```python
from build123d import *

# Parameters (mm, degrees)
F1_DEPTH = 1
F2_DEPTH = 13


with BuildPart() as f1:
    # F0 (on Top) → F1 (new body)
    with BuildSketch(Plane.XY):
        Polygon((2.864766, 10.75), (-2.864766, 10.75), (-5.25, 8.360261), (-5.25, -10.75), (5.25, -10.75), (5.25, 8.360261), align=None)
        Polygon((-4.25, 7.9466), (-2.45, 9.75), (2.45, 9.75), (4.25, 7.9466), (4.25, -9.75), (-4.25, -9.75), align=None, mode=Mode.SUBTRACT)
        Polygon((2.45, 9.75), (-2.45, 9.75), (-4.25, 7.9466), (-4.25, -9.75), (4.25, -9.75), (4.25, 7.9466), align=None)
    extrude(amount=F1_DEPTH)

    # F0 (on Top) → F2 (join)
    with BuildSketch(Plane.XY):
        Polygon((2.864766, 10.75), (-2.864766, 10.75), (-5.25, 8.360261), (-5.25, -10.75), (5.25, -10.75), (5.25, 8.360261), align=None)
        Polygon((-4.25, 7.9466), (-2.45, 9.75), (2.45, 9.75), (4.25, 7.9466), (4.25, -9.75), (-4.25, -9.75), align=None, mode=Mode.SUBTRACT)
    extrude(amount=F2_DEPTH)


solid = f1.part
```
Source: CAD feature listing. Evaluate the final solid. Frame: model axes, mm. A direction names the side the tool comes from. Coordinates: 2 decimals unless noted, no trailing zeros. Loops run counter-clockwise (first coordinate to the right, second up) from the corner with the lowest first, then second, coordinate; pieces in that order, holes last. Notation, with made-up numbers: (50, 81.5) -> (80, 81.5) arc R20 cw to (80, 88.5) -> close; hole circle Ø3 at (88.25, -11). An arc over 180 degrees is marked (long way). One line per item, written item: value. Start each with the question number.
Q1. Section query C-C, the plane z = 9.25. Return the cut outline in (x, y), and give its area (3 significant figures).
Q2. Line query: line 1 along X through (y, z) = (4.5, 10); line 2 along Y through (x, z) = (-1, 11.5); line 3 along Z through (x, y) = (-1.25, 3.5). Output: solid intervals per line, ascending.
Q3. Section query D-D, the plane x = 4.5. Return the cut outline in (y, z).
Q4. Set-up query: faces 1 (the face through (0, 0, 1)), 2 (the face through (4.07, 9.54, 6.41)). Return all of +Z, -Z, +X, -X, +Y, -Y with unobstructed straight access to the full face (end or side cutting, diameter ignored); none if empty.
Q5. Section query B-B, the plane x = 1. Return the cut outline in (y, z), and give its area (3 significant figures).
Q6. Mould query, pull axis X, two halves, no side actions, for faces 3 (the face through (-4.04, 9.57, 6.41)), 4 (the face through (0, 9.75, 7)), 5 (the face through (0, 0, 0)). Classes: pulls with the +X half, pulls with the -X half, needs draft (parallel to the pull), parting line crosses it, or undercut.
Q7. Section query A-A, the plane y = 7.5. Return the cut outline in (x, z).
Results:
1. outline: (-5.25, -10.75) -> (5.25, -10.75) -> (5.25, 8.36) -> (2.86, 10.75) -> (-2.86, 10.75) -> (-5.25, 8.36) -> close; hole (-4.25, -9.75) -> (4.25, -9.75) -> (4.25, 7.95) -> (2.45, 9.75) -> (-2.45, 9.75) -> (-4.25, 7.95) -> close
1. area: 57.5 mm^2
2. line 1: -5.25 to -4.25, 4.25 to 5.25
2. line 2: -10.75 to -9.75, 9.75 to 10.75
2. line 3: 0 to 1
3. outline: (-10.75, 0) -> (9.11, 0) -> (9.11, 13) -> (-10.75, 13) -> close
4. face 1: +Z
4. face 2: +Z, -Z, +X, +Y
5. outline: (-10.75, 0) -> (10.75, 0) -> (10.75, 13) -> (9.75, 13) -> (9.75, 1) -> (-9.75, 1) -> (-9.75, 13) -> (-10.75, 13) -> close
5. area: 45.5 mm^2
6. face 3: pulls with the -X half
6. face 4: undercut
6. face 5: needs draft
7. outline: (-5.25, 0) -> (5.25, 0) -> (5.25, 13) -> (4.25, 13) -> (4.25, 1) -> (-4.25, 1) -> (-4.25, 13) -> (-5.25, 13) -> close
